```python
from build123d import *

# Parameters (mm, degrees)
BOSS_EXTRUDE1_DEPTH = 5.08
SKETCH3_R           = 5.08
BOSS_EXTRUDE3_DEPTH = 2.54
FILLET1_R           = 0.635
SKETCH4_R           = 3.048
CUT_EXTRUDE1_DEPTH  = 12.58766262
FILLET2_R           = 0.254
FILLET3_R           = 0.254


with BuildPart() as part:
    # Sketch1 → Boss-Extrude1 (new body)
    with BuildSketch(Plane.XY):
        Polygon((-5.715, 3.299556788), (-5.715, -3.299556788), (0, -6.599113577), (5.715, -3.299556788), (5.715, 3.299556788), (0, 6.599113577), align=None)
    extrude(amount=BOSS_EXTRUDE1_DEPTH)

    # Sketch3 → Boss-Extrude3 (add)
    with BuildSketch(Plane.XY.offset(5.08)):
        Circle(SKETCH3_R)
    extrude(amount=BOSS_EXTRUDE3_DEPTH)

    # Fillet1
    fillet1_edges = [part.edges().sort_by_distance(p)[0] for p in [
        (-5.08, 0, 7.62),
    ]]
    fillet(fillet1_edges, radius=FILLET1_R)

    # Sketch4 → Cut-Extrude1 (cut, through all)
    with BuildSketch(Plane.XY.offset(7.62)):
        Circle(SKETCH4_R)
    extrude(amount=-CUT_EXTRUDE1_DEPTH, mode=Mode.SUBTRACT)

    # Fillet2
    fillet2_edges = [part.edges().sort_by_distance(p)[0] for p in [
        (-3.048, 0, 0),
        (2.8575, 4.949335183, 0),
        (5.715, 0, 0),
        (2.8575, -4.949335183, 0),
        (-2.8575, -4.949335183, 0),
        (-5.715, 0, 0),
        (-2.8575, 4.949335183, 0),
    ]]
    fillet(fillet2_edges, radius=FILLET2_R)

    # Fillet3
    fillet3_edges = [part.edges().sort_by_distance(p)[0] for p in [
        (-2.8575, -4.949335183, 5.08),
        (2.8575, -4.949335183, 5.08),
        (5.715, 0, 5.08),
        (-5.08, 0, 5.08),
        (2.8575, 4.949335183, 5.08),
        (-2.8575, 4.949335183, 5.08),
        (-5.715, 0, 5.08),
    ]]
    fillet(fillet3_edges, radius=FILLET3_R)


solid = part.part
```
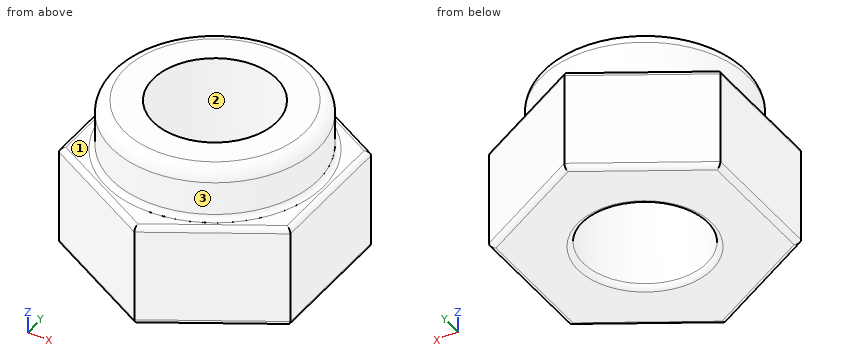
Work out the finished part from the listing and answer in its coordinate system (mm). Face numbers are marked on the shaded views. Give positions to 0.01 mm unless a question says otherwise; leave off trailing zeros. Loops run counter-clockwise (first coordinate to the right, second up) from the corner with the lowest first, then second, coordinate; pieces in that order, holes last. Notation, with made-up numbers: (24.25, 73) -> (80.25, 73) arc R14 cw to (80.25, 97) -> close; hole circle Ø9 at (0.5, 82). An arc over 180 degrees is marked (long way). One line per question, with ' | ' between items. Start each with the question number.
1) Section B-B, the plane z = 1.5 is taken. Determine the outline of the cut face in (x, y) (3 decimals).
2) Section C-C, the plane z = 6.5 is taken. Determine the outline of the cut face in (x, y).
3) Each of these flat-tipped pins is pushed along its axis until it touches: pin 1 (1.5 mm diameter, centred on x = 1.5, z = 5.5, fed in from -Y); pin 2 (2 mm diameter, centred on x = 3.5, y = 3, fed in from -Z); pin 3 (1.5 mm diameter, centred on x = 1, z = 5.5, fed in from -Y). Where does it stop, or does it pass through?
4) Section A-A, the plane y = 0 is taken. Determine the outline of the cut face in (x, z) (3 decimals).
5) Straight lines are drawn through the part: L1, parallel to Z at x = -4, y = 3.5; L2, parallel to Y at x = -2.75, z = 5.5; L3, parallel to Y at x = -0.5, z = 2.25. For each, find the intervals that lie inside material, in ascending order.
6) Determine the mould class of the marked faces 1, 2 and 3 for opening direction X: +X half, -X half, draft (parallel to the pull), parting line (faces both ways), or undercut.
Resolved:
1) outline: (-5.715, -3.3) -> (0, -6.599) -> (5.715, -3.3) -> (5.715, 3.3) -> (0, 6.599) -> (-5.715, 3.3) -> close; hole circle Ø6.096 at (0, 0)
2) outline: circle Ø10.16 at (0, 0); hole circle Ø6.1 at (0, 0)
3) pin 1: y = -5.99 | pin 2: z = 0 | pin 3: y = -6.28
4) outline: (-5.715, 0.254) arc R0.254 ccw to (-5.461, 0) -> (-3.302, 0) arc R0.254 ccw to (-3.048, 0.254) -> (-3.048, 7.62) -> (-4.445, 7.62) arc R0.635 ccw to (-5.08, 6.985) -> (-5.08, 5.334) arc R0.254 cw to (-5.334, 5.08) -> (-5.461, 5.08) arc R0.254 ccw to (-5.715, 4.826) -> close; (3.048, 0.254) arc R0.254 ccw to (3.302, 0) -> (5.461, 0) arc R0.254 ccw to (5.715, 0.254) -> (5.715, 4.826) arc R0.254 ccw to (5.461, 5.08) -> (5.334, 5.08) arc R0.254 cw to (5.08, 5.334) -> (5.08, 6.985) arc R0.635 ccw to (4.445, 7.62) -> (3.048, 7.62) -> close
5) L1: 0 to 5.08 | L2: -4.27 to -1.31, 1.31 to 4.27 | L3: -6.31 to -3.01, 3.01 to 6.31
6) face 1: draft | face 2: undercut | face 3: parting line
